Geometry check sheet. Reference: the model listing, model coordinates, mm. A direction names the side the tool comes from. Give positions to 0.01 mm unless a question says otherwise; leave off trailing zeros. Write each loop counter-clockwise with the first axis right and the second up, starting at its lowest first coordinate (ties: lowest second). Pieces come first, ordered by that corner, then holes. Notation, with made-up numbers: M 32,18.5 L 58,18.5 A24 ccw 58,53.5 Z; hole C -16.5,-22.5 d1. An arc over 180 degrees is marked long. One line per item, written item: value. Start each with the question number.
1. Gauge pin test, flat ends, axial feed: pin 1 (12.5 mm diameter, centred on x = 4.5, z = 30, fed in from +Y); pin 2 (5 mm diameter, centred on x = -1.5, z = 22.5, fed in from -Y); pin 3 (8 mm diameter, centred on y = 7, z = 22, fed in from -X); pin 4 (1.5 mm diameter, centred on y = 21.5, z = 10, fed in from -X). Record the tip position at first contact, or that the pin passes through.
2. Cross-section at C-C on y = 1. Record the cut outline in (x, z).
3. Cross-section at B-B on x = 19. Record the cut outline in (y, z), then the cut area to 3 significant figures.
4. Cross-section at D-D on y = 43.5. Record the cut outline in (x, z).
5. Scan lines: line 1 (Y direction, x = 1, z = 8); line 2 (Y direction, x = 2, z = 33); line 3 (X direction, y = 13, z = 12.5). Record each from-to range of solid material in increasing order.
6. Tool access check on faces 4 (the face through (12, -11.984, 9)), 5 (the face through (0, -2.484, 21)), 6 (the face through (1.967, 42.742, 38.395)), 7 (the face through (-9.822, -9.449, 34.376)), 8 (the face through (-1, 51.516, 21)). Record the directions out of +Z, -Z, +X, -X, +Y, -Y that give a thin tool (end or side, any length) a straight path to the whole face; none if there is none.
7. Cross-section at A-A on z = 18. Record the cut outline in (x, y).
8. Release check for a two-part mould opening along X. For faces 1 (the face through (-4.047, 38, 21)), 2 (the face through (-1, 23.016, 21)), 3 (the face through (-13, -11.984, 9)) record: pulls with the +X half, pulls with the -X half, needs draft (parallel to the pull), parting line crosses it, or undercut.
from build123d import *

# Parameters (mm, degrees)
BOSS_EXTRUDE1_DEPTH = 42
SKETCH2_W           = 7
SKETCH2_H           = 26
BOSS_EXTRUDE2_DEPTH = 42
SKETCH3_R           = 5.15
CUT_EXTRUDE1_DEPTH  = 2
SKETCH4_R           = 3.25
BOSS_EXTRUDE3_DEPTH = 7
SKETCH5_W           = 48.75
SKETCH5_H           = 2
BOSS_EXTRUDE4_DEPTH = 42


with BuildPart() as part:
    # Sketch1 → Boss-Extrude1 (new body)
    with BuildSketch(Plane.XY):
        Polygon((-24.92211838, -2.484423676), (-24.92211838, -4.984423676), (23.82788162, -4.984423676), (23.82788162, -2.484423676), (2.95288162, 25.515576324), (-4.04711838, 25.515576324), align=None)
        Polygon((-21.803802026, -2.484423676), (-2.792641312, 23.015576324), (1.698404552, 23.015576324), (20.709565266, -2.484423676), align=None, mode=Mode.SUBTRACT)
    extrude(amount=BOSS_EXTRUDE1_DEPTH)

    # Sketch2 → Boss-Extrude2 (add)
    with BuildSketch(Plane.XY.offset(42)):
        with Locations((-0.54711838, 38.515576324)):
            Rectangle(SKETCH2_W, SKETCH2_H)
    extrude(amount=-BOSS_EXTRUDE2_DEPTH)

    # Sketch3 → Cut-Extrude1 (cut)
    with BuildSketch(Plane(origin=(2.95288162, 0, 0), x_dir=(0, 0, -1), z_dir=(1, 0, 0))):
        with Locations((-33.25, 42.515576324)):
            Circle(SKETCH3_R)
        with Locations((-8.75, 42.515576324)):
            Circle(SKETCH3_R)
    extrude(amount=-CUT_EXTRUDE1_DEPTH, mode=Mode.SUBTRACT)

    # Sketch4 → Boss-Extrude3 (add)
    with BuildSketch(Plane.XZ.offset(4.984423676)):
        with Locations((-12.92211838, 33.4)):
            Circle(SKETCH4_R)
        with Locations((11.87788162, 33.4)):
            Circle(SKETCH4_R)
        with Locations((11.87788162, 8.6)):
            Circle(SKETCH4_R)
        with Locations((-12.92211838, 8.6)):
            Circle(SKETCH4_R)
    extrude(amount=BOSS_EXTRUDE3_DEPTH)

    # Sketch5 → Boss-Extrude4 (add)
    with BuildSketch(Plane.XY.offset(42)):
        with Locations((-0.54711838, -5.984423676)):
            Rectangle(SKETCH5_W, SKETCH5_H)
    extrude(amount=-BOSS_EXTRUDE4_DEPTH)


solid = part.part
Report:
1. pin 1: stops at y = 51.52
1. pin 2: stops at y = -6.98
1. pin 3: stops at x = -20.83
1. pin 4: stops at x = -7.6
2. outline: M -22.32,0 L -19.21,0 L -19.21,42 L -22.32,42 Z; M 18.11,0 L 21.23,0 L 21.23,42 L 18.11,42 Z
3. outline: M -6.98,0 L -2.48,0 L -2.48,42 L -6.98,42 Z; M -0.19,0 L 3.99,0 L 3.99,42 L -0.19,42 Z
3. area: 365 mm^2
4. outline: M -4.05,0 L 2.95,0 L 2.95,3.69 L 0.95,3.69 L 0.95,13.81 L 2.95,13.81 L 2.95,28.19 L 0.95,28.19 L 0.95,38.31 L 2.95,38.31 L 2.95,42 L -4.05,42 Z
5. line 1: y = -6.98 to -2.48, 23.02 to 37.42, 47.61 to 51.52
5. line 2: y = -6.98 to -2.48, 22.61 to 37.37, 47.66 to 51.52
5. line 3: x = -13.38 to -10.26, 9.17 to 12.28
6. face 4: +Z, -Z, +X, -X, -Y
6. face 5: +Z, -Z
6. face 6: +X
6. face 7: -Y
6. face 8: +Z, -Z, +X, -X, +Y
7. outline: M -24.92,-6.98 L 23.83,-6.98 L 23.83,-2.48 L 2.95,25.52 L 2.95,51.52 L -4.05,51.52 L -4.05,25.52 L -24.92,-2.48 Z; hole M -21.8,-2.48 L 20.71,-2.48 L 1.7,23.02 L -2.79,23.02 Z
8. face 1: pulls with the -X half
8. face 2: undercut
8. face 3: needs draft
